Source: three-view drawing plus pictorial views. Frame: mm from the lowest corner of the part. Give positions to 0.01 mm unless a question says otherwise; leave off trailing zeros. Order: outer loops, then holes, each group sorted by start corner. A loop starts at its lowest first (then second) coordinate and runs counter-clockwise, first axis right, second up. Notation, with made-up numbers: (22, 36.5) - (56, 36.5) arc R28 cw to (56, 63.5) - close; hole circle Ø11 at (71.25, 21). An arc over 180 degrees is marked (long way). Answer in a Markdown table with one row per item. Add a question column.
1. Section query D-D on x = 439. Return loops of the section in (y, z).
2. Ray query, line 1 (X direction, y = 5.5, z = 67.5); line 2 (Z direction, x = 297.2, y = 2.75); line 3 (X direction, y = 4.25, z = 81). Return the intervals inside material, ascending. Write a range as [from, to].
3. Section query C-C on y = 3.5. Return loops of the section in (x, z), and give its area (3 significant figures).
4. Section query B-B on z = 67.5. Return loops of the section in (x, y).
5. Section query A-A on x = 297.2. Return loops of the section in (y, z).
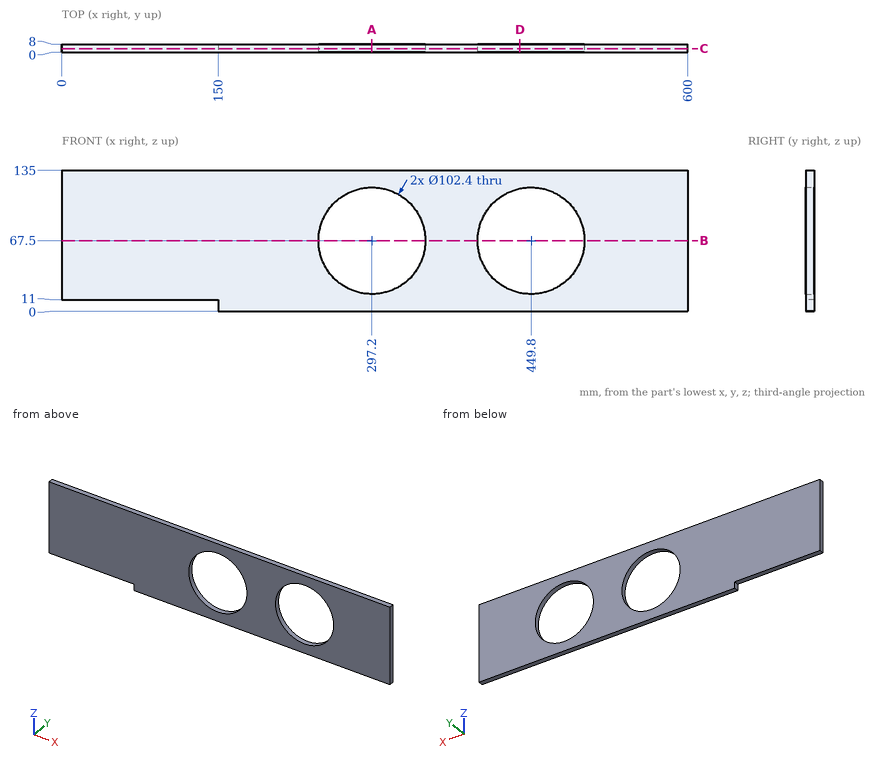
Answer:
| question | item | result |
|---|---|---|
| 1 | outline | (0, 0) - (8, 0) - (8, 17.45) - (0, 17.45) - close; (0, 117.55) - (8, 117.55) - (8, 135) - (0, 135) - close |
| 2 | line 1 | x = [0, 246], [348.4, 398.6], [501, 600] |
| 2 | line 2 | z = [0, 16.3], [118.7, 135] |
| 2 | line 3 | x = [0, 247.81], [346.59, 400.41], [499.19, 600] |
| 3 | outline | (0, 11) - (150, 11) - (150, 0) - (600, 0) - (600, 135) - (0, 135) - close; hole circle Ø102.4 at (297.2, 67.5); hole circle Ø102.4 at (449.8, 67.5) |
| 3 | area | 62,900 mm² |
| 4 | outline | (0, 0) - (246, 0) - (246, 8) - (0, 8) - close; (348.4, 0) - (398.6, 0) - (398.6, 8) - (348.4, 8) - close; (501, 0) - (600, 0) - (600, 8) - (501, 8) - close |
| 5 | outline | (0, 0) - (8, 0) - (8, 16.3) - (0, 16.3) - close; (0, 118.7) - (8, 118.7) - (8, 135) - (0, 135) - close |
